Model file for the job. Use its own axes, mm. Give positions to 0.01 mm unless a question says otherwise; leave off trailing zeros. Loops run counter-clockwise (first coordinate to the right, second up) from the corner with the lowest first, then second, coordinate; pieces in that order, holes last. Notation, with made-up numbers: M 66.25,54.25 L 93.25,54.25 A13 cw 93.25,73.25 Z; hole C 46,85.25 d6. An arc over 180 degrees is marked long. Answer in a Markdown table with one row per item.
```python
from build123d import *

# Parameters (mm, degrees)
F3_R = 3


with BuildPart() as f2:
    # F0 (on Front) → F2 (revolve)
    with BuildSketch(Plane.XZ):
        with BuildLine():
            ThreePointArc((2.540189, -25.569025), (2.830894, -18.423916), (6.156331, -12.093151))
            ThreePointArc((6.156331, -12.093151), (21.682175, 17.25035), (23.329504, 50.407239))
            Line((23.329504, 50.407239), (21.850841, 50.15514))
            ThreePointArc((21.850841, 50.15514), (20.235781, 17.647775), (5.014079, -11.120906))
            ThreePointArc((5.014079, -11.120906), (2.62263, -12.203154), (0, -12.093151))
            Line((0, -12.093151), (0, -75.33066))
            Line((0, -75.33066), (28.07332, -75.33066))
            Line((28.07332, -75.33066), (28.07332, -71.624145))
            Line((28.07332, -71.624145), (10.141856, -71.624145))
            ThreePointArc((10.141856, -71.624145), (4.882403, -67.064973), (2.878637, -60.399178))
            Line((2.878637, -60.399178), (2.540189, -25.569025))
        make_face()
    revolve(axis=Axis((0, 0, 7.113926), (0, 0, -1)))

    # F3
    f3_edges = [f2.edges().sort_by_distance(p)[0] for p in [
        (-28.07332, 0, -71.624145),
    ]]
    fillet(f3_edges, radius=F3_R)


solid = f2.part
```
(1) Mould opens along Z. For faces 1 (the flat face through (0, 0, -75.331)), 2 (the cylindrical face through (-22.28, 17.08, -74.97)), 3 (the conical face through (2.582, -0.813, -42.74)) say: pulls with the +Z half, pulls with the -Z half, needs draft (parallel to the pull), parting line crosses it, or undercut.
Established:
| item | result |
|---|---|
| face 1 | pulls with the -Z half |
| face 2 | needs draft |
| face 3 | undercut |
(2) Wall check: L1, parallel to Y at x = -4.5, z = -3.5; L2, parallel to Y at x = 21, z = 44.5; L3, parallel to X at y = 4, z = 22. Give the ranges that are in metal, low to high.
Established:
| item | result |
|---|---|
| L1 | y = -11.65 to -9.72, 9.72 to 11.65 |
| L2 | y = -11.83 to -8.34, 8.34 to 11.83 |
| L3 | x = -22.47 to -20.91, 20.91 to 22.47 |
(3) Flat gauge pins, fed straight in: P1, Ø8, axis at x = -7, y = -19.5, coming from the +Z side; P2, Ø8, axis at x = -1.5, z = 7.5, coming from the +Y side; P3, Ø1.5, axis at y = 9, z = 20, coming from the -X side; P4, Ø5, axis at x = -1.5, z = 1, coming from the -Y side. Where does each tip first touch, or does it go through?
Established:
| item | result |
|---|---|
| P1 | stops at z = 50.41 |
| P2 | stops at y = 19.82 |
| P3 | stops at x = -20.86 |
| P4 | stops at y = -16.38 |
(4) Saw through at A-A, the plane z = -48. Give the cut face in (x, y).
Established:
| item | result |
|---|---|
| outline | C 0,0 d5.52 |
